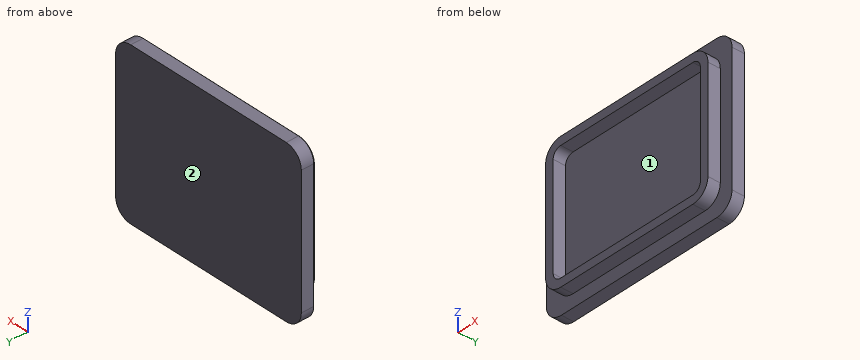
```python
from build123d import *

# Parameters (mm, degrees)
SKETCH1_W           = 62.484
SKETCH1_H           = 49.784
BOSS_EXTRUDE1_DEPTH = 3.81
SKETCH2_W           = 54.61
SKETCH2_H           = 41.91
SKETCH2_W_2         = 49.53
SKETCH2_H_2         = 36.83
BOSS_EXTRUDE3_DEPTH = 3.81
FILLET1_R           = 5.08
FILLET2_R           = 5.08
FILLET3_R           = 2.54


with BuildPart() as part:
    # Sketch1 → Boss-Extrude1 (new body)
    with BuildSketch(Plane(origin=(0, 0, 0), x_dir=(1, 0, 0), z_dir=(0, 1, 0))):
        with Locations((31.242, -24.892)):
            Rectangle(SKETCH1_W, SKETCH1_H)
    extrude(amount=BOSS_EXTRUDE1_DEPTH)

    # Sketch2 → Boss-Extrude3 (add)
    with BuildSketch(Plane.XZ):
        with Locations((31.242, 24.892)):
            Rectangle(SKETCH2_W, SKETCH2_H)
        with Locations((31.242, 24.892)):
            Rectangle(SKETCH2_W_2, SKETCH2_H_2, mode=Mode.SUBTRACT)
    extrude(amount=BOSS_EXTRUDE3_DEPTH)

    # Fillet1
    fillet1_edges = [part.edges().sort_by_distance(p)[0] for p in [
        (0, 1.905, 49.784),
        (0, 1.905, 0),
        (62.484, 1.905, 0),
        (62.484, 1.905, 49.784),
    ]]
    fillet(fillet1_edges, radius=FILLET1_R)

    # Fillet2
    fillet2_edges = [part.edges().sort_by_distance(p)[0] for p in [
        (58.547, -1.905, 3.937),
        (58.547, -1.905, 45.847),
        (3.937, -1.905, 45.847),
        (3.937, -1.905, 3.937),
    ]]
    fillet(fillet2_edges, radius=FILLET2_R)

    # Fillet3
    fillet3_edges = [part.edges().sort_by_distance(p)[0] for p in [
        (56.007, -1.905, 43.307),
        (6.477, -1.905, 43.307),
        (6.477, -1.905, 6.477),
        (56.007, -1.905, 6.477),
    ]]
    fillet(fillet3_edges, radius=FILLET3_R)


solid = part.part
```
Geometry check sheet. Reference: the model listing, model coordinates, mm. Face numbers are marked on the shaded views. Give positions to 0.01 mm unless a question says otherwise; leave off trailing zeros. Write each loop counter-clockwise with the first axis right and the second up, starting at its lowest first coordinate (ties: lowest second). Pieces come first, ordered by that corner, then holes.
1) Release check for a two-part mould opening along Z. For the marked faces 1 and 2 record: pulls with the +Z half, pulls with the -Z half, needs draft (parallel to the pull), parting line crosses it, or undercut.
2) Section check C-C, the plane z = 24.5. Record the boundary of the cut face in (x, y).
3) Material ranges on L1, parallel to X at y = -0.75, z = 31.5; L2, parallel to Z at x = 16, y = -2.75; L3, parallel to Y at x = 12.5, z = 39.5, recorded low to high.
4) Gauge pin test, flat ends, axial feed: pin 1 (1.1 mm diameter, centred on x = 22.5, y = -2, fed in from -Z); pin 2 (2 mm diameter, centred on y = -2.5, z = 36, fed in from -X); pin 3 (18.5 mm diameter, centred on x = 36.5, z = 19, fed in from -Y). Record the tip position at first contact, or that the pin passes through.
5) Section check A-A, the plane y = -1. Record the boundary of the cut face in (x, z).
6) Section check B-B, the plane x = 15. Record the boundary of the cut face in (y, z).
Computed:
1. face 1: undercut
1. face 2: needs draft
2. outline: (0, 0) - (3.94, 0) - (3.94, -3.81) - (6.48, -3.81) - (6.48, 0) - (56.01, 0) - (56.01, -3.81) - (58.55, -3.81) - (58.55, 0) - (62.48, 0) - (62.48, 3.81) - (0, 3.81) - close
3. L1: x = 3.94 to 6.48, 56.01 to 58.55
3. L2: z = 3.94 to 6.48, 43.31 to 45.85
3. L3: y = 0 to 3.81
4. pin 1: stops at z = 3.94
4. pin 2: stops at x = 3.94
4. pin 3: stops at y = 0
5. outline: (3.94, 9.02) arc R5.08 ccw to (9.02, 3.94) - (53.47, 3.94) arc R5.08 ccw to (58.55, 9.02) - (58.55, 40.77) arc R5.08 ccw to (53.47, 45.85) - (9.02, 45.85) arc R5.08 ccw to (3.94, 40.77) - close; hole (6.48, 9.02) arc R2.54 ccw to (9.02, 6.48) - (53.47, 6.48) arc R2.54 ccw to (56.01, 9.02) - (56.01, 40.77) arc R2.54 ccw to (53.47, 43.31) - (9.02, 43.31) arc R2.54 ccw to (6.48, 40.77) - close
6. outline: (-3.81, 3.94) - (0, 3.94) - (0, 0) - (3.81, 0) - (3.81, 49.78) - (0, 49.78) - (0, 45.85) - (-3.81, 45.85) - (-3.81, 43.31) - (0, 43.31) - (0, 6.48) - (-3.81, 6.48) - close
